from build123d import *

# Parameters (mm, degrees)
F1_R     = 17.4
F2_DEPTH = 6
F4_COUNT = 18


with BuildPart() as f2:
    # F1 (on Top) + F0 (on Top) → F2 (new body)
    with BuildSketch(Plane.XY):
        Circle(F1_R)
    with BuildSketch(Plane.XY):
        Polygon((-1.046719, 19.972591), (-2.271156, 17.251141), (2.271156, 17.251141), (1.046719, 19.972591), (0, 19.972591), align=None)
    extrude(amount=F2_DEPTH)

    # F4: F2 ×18 about axis
    f4_axis = Axis((0, 0, 1.5), (0, 0, 1))


with BuildPart() as f2_1:
    add(f2.part)
    for i in range(1, F4_COUNT):
        add(f2.part.rotate(f4_axis, i * 360 / F4_COUNT))


solid = f2_1.part
Design review of the part built by this model. Coordinates are the model's own, in mm. A direction names the side the tool comes from. Give positions to 0.01 mm unless a question says otherwise; leave off trailing zeros. Order: outer loops, then holes, each group sorted by start corner. A loop starts at its lowest first (then second) coordinate and runs counter-clockwise, first axis right, second up.
1. Mouldability with a two-part tool opening along X and no side actions: class faces 5 (the flat face through (0, 0, 0)), 6 (the flat face through (6.82, -18.77, 2.96)), 7 (the flat face through (4.79, -18.04, 2.96)), 8 (the flat face through (-19.672, -3.454, 2.958)) as +X half, -X half, draft (parallel to the pull), parting line (faces both ways), or undercut.
Solution:
face 5: draft
face 6: +X half
face 7: undercut
face 8: -X half
2. For pin 1 Ø3 at (x, y) = (-12.5, 4.5) entering from -Z; pin 2 Ø2 at (x, z) = (8.5, 5) entering from -Y; pin 3 Ø1.5 at (y, z) = (-8.5, 3.5) entering from +X; pin 4 Ø1.5 at (x, z) = (-12, 5.5) entering from +Y, all flat-tipped, find the tip position at first contact; note any pin that passes through.
Solution:
pin 1: stops at z = 0
pin 2: stops at y = -18.52
pin 3: stops at x = 17.82
pin 4: stops at y = 15.97
3. To check wall thickness, follow L1, parallel to X at y = 15.5, z = 1.8; L2, parallel to X at y = 0, z = 4.35; L3, parallel to X at y = -2.5, z = 5.35. State the ranges of each line that lie inside material, in increasing order.
Solution:
L1: x = -12.6 to -11.06, -8.03 to 8.03, 11.06 to 12.6
L2: x = -17.4 to 17.4
L3: x = -19.84 to 19.84
4. Tool access review of faces 1 (the cylindrical face through (-3.032, -17.134, 2.958)), 2 (the cylindrical face through (-16.354, -5.941, 2.958)), 3 (the flat face through (-15.27, 10.74, 2.96)), 4 (the cylindrical face through (-13.322, 11.193, 2.958)): name each direction out of +Z, -Z, +X, -X, +Y, -Y from which nothing blocks a thin tool from reaching the whole face with its end or side.
Solution:
face 1: +Z, -Z, -Y
face 2: +Z, -Z, -X
face 3: +Z, -Z, +Y
face 4: +Z, -Z
5. Add section B-B, the plane x = -6.5. State the section outline as (y, z) points, then the cut area to 3 significant figures.
Solution:
outline: (-18.89, 0) - (18.89, 0) - (18.89, 6) - (-18.89, 6) - close
area: 227 mm2
6. Add section C-C, the plane y = -16.5. State the section outline as (x, z) points, then the cut area to 3 significant figures.
Solution:
outline: (-7.96, 0) - (7.96, 0) - (7.96, 6) - (-7.96, 6) - close
area: 95.5 mm2
